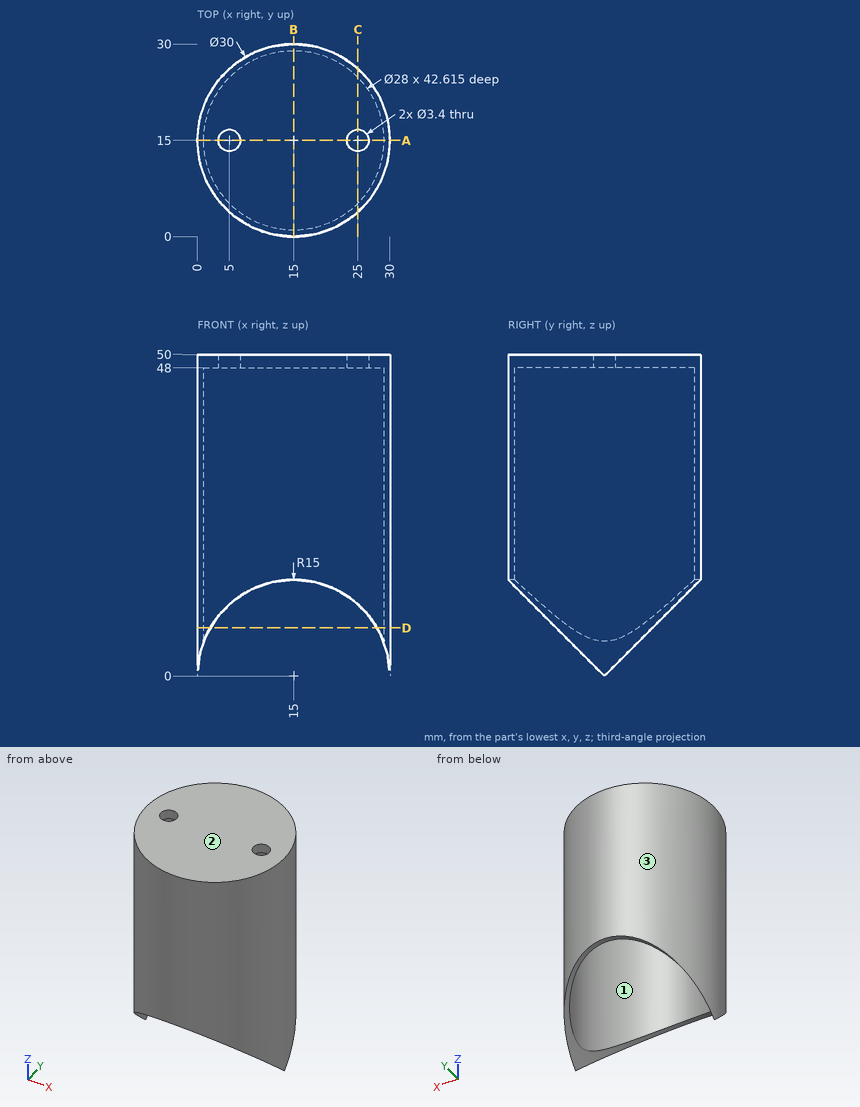
Part print with two shaded views. Sizes in mm from the minimum x, y, z corner. Round coordinates to 2 decimals unless told otherwise and drop trailing zeros. Order: outer loops, then holes, each group sorted by start corner. A loop starts at its lowest first (then second) coordinate and runs counter-clockwise, first axis right, second up. Notation, with made-up numbers: (1, 57.5) - (24, 57.5) arc R22 ccw to (24, 82.5) - close; hole circle Ø3 at (61.25, -18.5). An arc over 180 degrees is marked (long way). Answer in a Markdown table with one row per item. Add a question column.
(1) Probe L1, parallel to X at y = 15, z = 48.5; L2, parallel to Y at x = 15, z = 31. List the from-to ranges inside material, lowest first. Write a range as [from, to].
(2) Mould opens along Y. For the marked faces 1, 2 and 3 say: +Y half, -Y half, draft (parallel to the pull), parting line (faces both ways), or undercut.
(3) Drop flat-ended pins along their axis: pin 1 Ø6 at (x, z) = (11, 42.5) entering from -Y; pin 2 Ø6 at (x, z) = (5, 26.5) entering from +Y; pin 3 Ø8 at (x, y) = (26, 23) entering from -Z; pin 4 Ø2 at (x, y) = (5, 15) entering from +Z. Give the stop position or say it passes through.
(4) Band-saw the part on C-C on x = 25. List the corners of the cut face in (y, z).
(5) Band-saw the part on B-B on x = 15. List the corners of the cut face in (y, z), and give its area (3 significant figures).
(6) Band-saw the part on A-A on y = 15. List the corners of the cut face in (x, z) (1 decimal), and give its area (3 significant figures).
(7) Band-saw the part on D-D on z = 7.5. List the corners of the cut face in (x, y), and give its area (3 significant figures).
Data:
| question | item | result |
|---|---|---|
| 1 | L1 | x = [0, 3.3], [6.7, 23.3], [26.7, 30] |
| 1 | L2 | y = [0, 1], [29, 30] |
| 2 | face 1 | undercut |
| 2 | face 2 | draft |
| 2 | face 3 | parting line |
| 3 | pin 1 | stops at y = 0.03 |
| 3 | pin 2 | stops at y = 28.27 |
| 3 | pin 3 | stops at z = 5.36 |
| 3 | pin 4 | passes through |
| 4 | outline | (3.82, 11.18) - (5.2, 11.18) - (5.2, 48) - (13.3, 48) - (13.3, 50) - (3.82, 50) - close; (16.7, 48) - (24.8, 48) - (24.8, 11.18) - (26.18, 11.18) - (26.18, 50) - (16.7, 50) - close |
| 5 | outline | (0, 15) - (1, 15) - (1, 48) - (29, 48) - (29, 15) - (30, 15) - (30, 50) - (0, 50) - close |
| 5 | area | 126 mm^2 |
| 6 | outline | (0, 0) arc R15 cw to (1, 5.4) - (1, 48) - (3.3, 48) - (3.3, 50) - (0, 50) - close; (6.7, 48) - (23.3, 48) - (23.3, 50) - (6.7, 50) - close; (26.7, 48) - (29, 48) - (29, 5.4) arc R15 cw to (30, 0) - (30, 50) - (26.7, 50) - close |
| 6 | area | 135 mm^2 |
| 7 | outline | (2.01, 7.5) - (2.01, 9.78) arc R14 cw to (2.01, 20.22) - (2.01, 22.5) arc R15 ccw to start; (27.99, 7.5) arc R15 ccw to (27.99, 22.5) - (27.99, 20.22) arc R14 cw to (27.99, 9.78) - close |
| 7 | area | 26.6 mm^2 |
